from build123d import *

# Parameters (mm, degrees)
SKETCH1_R           = 2.5
BOSS_EXTRUDE2_DEPTH = 10


with BuildPart() as part:
    # Sketch1 → Boss-Extrude2 (new body)
    with BuildSketch(Plane(origin=(0, 0, 0), x_dir=(1, 0, 0), z_dir=(0, 1, 0))):
        with BuildLine():
            ThreePointArc((90, 5), (95, 0), (90, -5))
            Line((90, -5), (-90, -5))
            Line((-90, -5), (-90, 5))
            Line((-90, 5), (90, 5))
        make_face()
        with Locations(Location((90, 0, 0), (0, 0, 270))):
            Circle(SKETCH1_R, mode=Mode.SUBTRACT)
    extrude(amount=BOSS_EXTRUDE2_DEPTH)

    # Sketch6 → Revolve2 (revolve)
    with BuildSketch(Plane.XY, mode=Mode.PRIVATE) as revolve2_sk:
        Polygon((-88.175, 0), (-78.65, 12.7), (-83.65, 12.7), (-93.175, 0), align=None)
    revolve(revolve2_sk.sketch.rotate(Axis((-99.525, 14.826221604, 0), (0, -1, 0)), 90), axis=Axis((-99.525, 14.826221604, 0), (0, -1, 0)))

    # Sketch7 → Cut-Revolve1 (revolve, cut)
    with BuildSketch(Plane.XY):
        Polygon((-83.65, 12.7), (-93.175, 0), (-99.525, 0), (-99.525, 12.7), align=None)
    revolve(axis=Axis((-99.525, 12.7, 0), (0, -1, 0)), mode=Mode.SUBTRACT)


solid = part.part
Design review of the part built by this model. Coordinates are the model's own, in mm. Coordinates: 2 decimals unless noted, no trailing zeros. Order: outer loops, then holes, each group sorted by start corner. A loop starts at its lowest first (then second) coordinate and runs counter-clockwise, first axis right, second up. Notation, with made-up numbers: (61.25, 76.5) -> (65.25, 76.5) arc R27 ccw to (65.25, 93.5) -> close; hole circle Ø5 at (-12, 32.5). An arc over 180 degrees is marked (long way). One line per item, written item: value.
1) Clearance check with flat-ended pins moving along their axes: P1, Ø3, axis at x = 39.5, y = 7, coming from the +Z side; P2, Ø1.5, axis at y = 6.5, z = -15, coming from the +X side; P3, Ø10, axis at x = -59, z = -6.5, coming from the +Y side. State where each tip first meets the part, or that it passes through.
Output values:
P1: stops at z = 5
P2: stops at x = -91.34
P3: stops at y = 10
2) We need section A-A, the plane z = 0. Give the boundary of the cut face in (x, y) (3 decimals).
Output values:
outline: (-120.4, 12.7) -> (-110.875, 0) -> (-105.875, 0) -> (-115.4, 12.7) -> close; (-93.175, 0) -> (87.5, 0) -> (87.5, 10) -> (-80.675, 10) -> (-78.65, 12.7) -> (-83.65, 12.7) -> close; (92.5, 0) -> (95, 0) -> (95, 10) -> (92.5, 10) -> close
3) We need section C-C, the plane x = 36. Give the boundary of the cut face in (y, z), then the cut area to 3 significant figures.
Output values:
outline: (0, -5) -> (10, -5) -> (10, 5) -> (0, 5) -> close
area: 100 mm2
4) To check wall thickness, follow probe 1 along X at (y, z) = (5.75, 0); probe 2 along X at (y, z) = (1, -1); probe 3 along Z at (x, y) = (-80, 8.25). State the ranges of each line that lie inside material, in increasing order. Write a range as [from, to].
Output values:
probe 1: x = [-115.19, -110.19], [-88.86, 87.5], [92.5, 95]
probe 2: x = [-111.58, -106.55], [-92.5, 87.71], [92.29, 94.9]
probe 3: z = [-5, 5]
5) Draft analysis for pull direction Z (two halves, no side actions). For faces 1 (the face through (92.48, 4.93, -0.33)), 2 (the face through (2, 5, 5)), 3 (the face through (95, 5, 0)), 4 (the face through (-1, 5, -5)), state which applies: +Z half, -Z half, draft (parallel to the pull), parting line (faces both ways), or undercut.
Output values:
face 1: undercut
face 2: +Z half
face 3: parting line
face 4: -Z half
6) We need section B-B, the plane y = 7.25. Give the boundary of the cut face in (x, z) (1 decimal).
Output values:
outline: (-83.5, -5) -> (90, -5) arc R5 ccw to (90, 5) -> (-83.5, 5) arc R16.8 ccw (long way) to start; hole circle Ø23.6 at (-99.5, 0); hole circle Ø5 at (90, 0)
